Build history of the part. All positions in model axes, mm. A direction names the side the tool comes from. Round coordinates to 2 decimals unless told otherwise and drop trailing zeros. Write each loop counter-clockwise with the first axis right and the second up, starting at its lowest first coordinate (ties: lowest second). Pieces come first, ordered by that corner, then holes.
from build123d import *

# Parameters (mm, degrees)
F0_W      = 115
F0_H      = 170
F1_DEPTH  = 4
F2_W      = 110.5
F2_H      = 166
F3_DEPTH  = 1.5
F4_W      = 98.5
F4_H      = 154
F5_DEPTH  = 2.501
F7_W      = 6
F7_H      = 6
F8_DEPTH  = 2.5
F9_R      = 3
F10_DEPTH = 2.501
F11_R     = 2
F12_R     = 2
F13_R     = 1.5


with BuildPart() as f1:
    # F0 (on Top) → F1 (new body)
    with BuildSketch(Plane.XY):
        Rectangle(F0_W, F0_H)
    extrude(amount=F1_DEPTH)

    # F2 (on face) → F3 (cut)
    with BuildSketch(Plane(origin=(0, 0, 0), x_dir=(1, 0, 0), z_dir=(0, 0, -1))):
        Rectangle(F2_W, F2_H)
    extrude(amount=-F3_DEPTH, mode=Mode.SUBTRACT)

    # F4 (on face) → F5 (cut, through all)
    with BuildSketch(Plane(origin=(0, 0, 1.5), x_dir=(1, 0, 0), z_dir=(0, 0, -1))):
        Rectangle(F4_W, F4_H)
    extrude(amount=-F5_DEPTH, mode=Mode.SUBTRACT)

    # F7 (on face) → F8 (join, through all)
    with BuildSketch(Plane(origin=(0, 0, 1.5), x_dir=(1, 0, 0), z_dir=(0, 0, -1))):
        with Locations((46.25, -74)):
            Rectangle(F7_W, F7_H)
        with Locations((-46.25, -74)):
            Rectangle(F7_W, F7_H)
        with Locations((-46.25, 74)):
            Rectangle(F7_W, F7_H)
        with Locations((46.25, 74)):
            Rectangle(F7_W, F7_H)
    extrude(amount=-F8_DEPTH)

    # F9 (on face) → F10 (cut, through all)
    with BuildSketch(Plane(origin=(0, 0, 1.5), x_dir=(1, 0, 0), z_dir=(0, 0, -1))):
        with Locations((49.75, -77.5)):
            Circle(F9_R)
        with Locations((-49.75, -77.5)):
            Circle(F9_R)
        with Locations((-49.75, 77.5)):
            Circle(F9_R)
        with Locations((49.75, 77.5)):
            Circle(F9_R)
    extrude(amount=-F10_DEPTH, mode=Mode.SUBTRACT)

    # F11
    f11_edges = [f1.edges().sort_by_distance(p)[0] for p in [
        (-43.25, 77, 2.75),
        (-43.25, 71, 2.75),
        (-49.25, 71, 2.75),
        (49.25, 71, 2.75),
        (43.25, 71, 2.75),
        (43.25, 77, 2.75),
        (49.25, -71, 2.75),
        (43.25, -71, 2.75),
        (43.25, -77, 2.75),
        (-43.25, -77, 2.75),
        (-43.25, -71, 2.75),
        (-49.25, -71, 2.75),
    ]]
    fillet(f11_edges, radius=F11_R)

    # F12
    f12_edges = [f1.edges().sort_by_distance(p)[0] for p in [
        (-57.5, 85, 2),
        (57.5, 85, 2),
        (57.5, -85, 2),
        (-57.5, -85, 2),
    ]]
    fillet(f12_edges, radius=F12_R)

    # F13
    f13_edges = [f1.edges().sort_by_distance(p)[0] for p in [
        (55.25, 83, 0.75),
        (-55.25, 83, 0.75),
        (-55.25, -83, 0.75),
        (55.25, -83, 0.75),
    ]]
    fillet(f13_edges, radius=F13_R)


solid = f1.part
1) Mould opens along Y. For faces 1 (the flat face through (-1, -85, 2)), 2 (the flat face through (-57.5, -1, 2)), 3 (the cylindrical face through (-52.131, 79.325, 2.732)) say: released by +Y, released by -Y, zero draft, split by the parting line, or undercut.
Results:
face 1: released by -Y
face 2: zero draft
face 3: undercut
2) Wall check: L1, parallel to X at y = -77.5, z = 2.15; L2, parallel to Y at x = 49.75, z = 2.85; L3, parallel to Y at x = -5, z = 1.3. Give the ranges that are in metal, low to high.
Results:
L1: x = -57.5 to -52.75, -46.75 to 46.75, 52.75 to 57.5
L2: y = -85 to -80.5, -74.5 to 74.5, 80.5 to 85
L3: y = -85 to -83, 83 to 85
3) Slice it at B-B (z = 0.6). Write the cut outline in (x, y), plus the area to 3 significant figures.
Results:
outline: (-57.5, -83) arc R2 ccw to (-55.5, -85) - (55.5, -85) arc R2 ccw to (57.5, -83) - (57.5, 83) arc R2 ccw to (55.5, 85) - (-55.5, 85) arc R2 ccw to (-57.5, 83) - close; hole (-55.25, -81.5) arc R1.5 ccw to (-53.75, -83) - (53.75, -83) arc R1.5 ccw to (55.25, -81.5) - (55.25, 81.5) arc R1.5 ccw to (53.75, 83) - (-53.75, 83) arc R1.5 ccw to (-55.25, 81.5) - close
area: 1,210 mm2
4) Slice it at C-C (x = -29). Write the cut outline in (y, z).
Results:
outline: (-85, 0) - (-83, 0) - (-83, 1.5) - (-77, 1.5) - (-77, 4) - (-85, 4) - close; (77, 1.5) - (83, 1.5) - (83, 0) - (85, 0) - (85, 4) - (77, 4) - close
5) Slice it at A-A (y = 26.5). Write the cut outline in (x, z), plus the area to 3 significant figures.
Results:
outline: (-57.5, 0) - (-55.25, 0) - (-55.25, 1.5) - (-49.25, 1.5) - (-49.25, 4) - (-57.5, 4) - close; (49.25, 1.5) - (55.25, 1.5) - (55.25, 0) - (57.5, 0) - (57.5, 4) - (49.25, 4) - close
area: 48.0 mm2
6) Which spindle directions (+Z, -Z, +X, -X, +Y, -Y) get a long thin tool onto all of the face, cutting with end or side? Do faces 4 (the flat face through (57.5, -1, 2)), 5 (the flat face through (-53, 0, 1.5)). Say none if no direction does.
Results:
face 4: +Z, -Z, +X, +Y, -Y
face 5: -Z
7) Pin check, flat tip, straight feed: pin 1 Ø9.5 at (x, y) = (49.75, -77.5) entering from -Z. Stop position of the tip, or through.
Results:
pin 1: stops at z = 1.5
